The drawing under review shows one solid part. Ordinate dimensions are in mm from its lowest x, y, z. Round coordinates to 2 decimals unless told otherwise and drop trailing zeros. Order: outer loops, then holes, each group sorted by start corner. A loop starts at its lowest first (then second) coordinate and runs counter-clockwise, first axis right, second up. Notation, with made-up numbers: M -35.5,6.25 L -30.5,6.25 A26 cw -30.5,41.25 Z; hole C -21,66 d4. An arc over 180 degrees is marked long. Answer as a JSON object with one key per item and string values. Group by question number.
1) Consider section B-B, the plane z = 3.5. Write out the cut boundary in (x, y), then the cut area to 3 significant figures.
2) Insertion check: pin 1 Ø4 at (x, z) = (52, 44) entering from -Y. The pin has a flat end and moves straight along its axis. Give the tip position at first contact, or say it passes through.
3) Consider section A-A, the plane x = 3.5. Write out the cut boundary in (y, z), then the cut area to 3 significant figures.
4) To check wall thickness, follow line 1 (Z direction, x = 61.5, y = 0.4); line 2 (X direction, y = 0.6, z = 52.5); line 3 (X direction, y = 0.15, z = 53). State the ranges of each line that lie inside material, in increasing order.
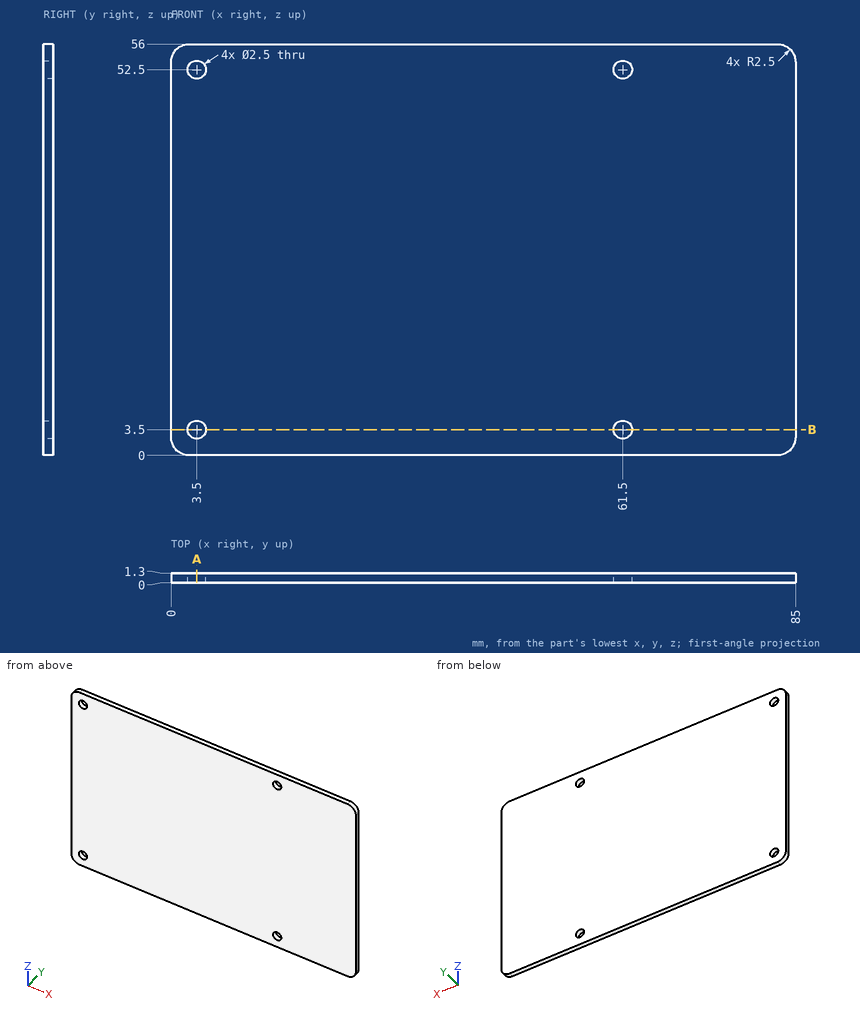
Results list:
{
 "1": {"outline": "M 0,0 L 2.25,0 L 2.25,1.3 L 0,1.3 Z; M 4.75,0 L 60.25,0 L 60.25,1.3 L 4.75,1.3 Z; M 62.75,0 L 85,0 L 85,1.3 L 62.75,1.3 Z", "area": "104 mm^2"},
 "2": {"pin 1": "y = 0"},
 "3": {"outline": "M 0,0 L 1.3,0 L 1.3,2.25 L 0,2.25 Z; M 0,4.75 L 1.3,4.75 L 1.3,51.25 L 0,51.25 Z; M 0,53.75 L 1.3,53.75 L 1.3,56 L 0,56 Z", "area": "66.3 mm^2"},
 "4": {"line 1": "0 to 2.25, 4.75 to 51.25, 53.75 to 56", "line 2": "0 to 2.25, 4.75 to 60.25, 62.75 to 85", "line 3": "0 to 2.35, 4.65 to 60.35, 62.65 to 85"}
}
